Can you work these out from the model? Positions are in its coordinate system, mm. A direction names the side the tool comes from. Round coordinates to 2 decimals unless told otherwise and drop trailing zeros. Order: outer loops, then holes, each group sorted by start corner. A loop starts at its lowest first (then second) coordinate and runs counter-clockwise, first axis right, second up.
Q1. Will these pins go through, and if not, where does the flat tip stop? P1, Ø6.5, axis at x = 3.5, z = -13.5, coming from the +Y side; P2, Ø2.5, axis at x = 9.5, z = -7, coming from the +Y side.
Q2. We'd pull the mould along Y, two halves only. Please class faces 4 (the face through (8, 2, -13)), 5 (the face through (6.2, 3.8, -13)), 6 (the face through (27.88, 0.57, -0.6)), 7 (the face through (34, 7, -25.03)): pulls with the +Y half, pulls with the -Y half, needs draft (parallel to the pull), parting line crosses it, or undercut.
Q3. If I drill on line 1 (X direction, y = 2.5, z = -5.25); line 2 (X direction, y = 5, z = -21.25); line 3 (X direction, y = 7, z = -11.25), over which ranges is the centre line in solid material (lowest first)?
Q4. For faces 1 (the face through (12.4, 5, -13)), 2 (the face through (4, 5.6, -13)), 3 (the face through (0, 3, -13)), which set-ups out of +Z, -Z, +X, -X, +Y, -Y let a thin tool reach every point of the face, with its end or its side?
Q5. If we section it at C-C (x = 31.5): Please give me the cut outline in (y, z), plus the area to 3 significant figures.
Q6. If we section it at D-D (z = -19.5): Please give me the cut outline in (x, y), plus the area to 3 significant figures.
Q7. If we section it at A-A (y = 3): Please give me the cut outline in (x, z).
from build123d import *

# Parameters (mm, degrees)
SKETCH1_W           = 55
SKETCH1_H           = 25.6
BOSS_EXTRUDE1_DEPTH = 7.6
CUT_EXTRUDE1_DEPTH  = 25.6
FILLET1_R           = 2


with BuildPart() as part:
    # Sketch1 → Boss-Extrude1 (new body)
    with BuildSketch(Plane(origin=(0, 0, 0), x_dir=(1, 0, 0), z_dir=(0, 1, 0))):
        with Locations((27.5, 12.8)):
            Rectangle(SKETCH1_W, SKETCH1_H)
    extrude(amount=BOSS_EXTRUDE1_DEPTH)

    # Sketch2 → Cut-Extrude1 (cut)
    with BuildSketch(Plane(origin=(0, 0, -25.6), x_dir=(-1, 0, 0), z_dir=(0, 0, -1))):
        Polygon((-8, 5.6), (-4.4, 2), (-12.4, 2), (-12.4, 7.6), (0, 7.6), (0, 5.6), align=None)
    extrude(amount=-CUT_EXTRUDE1_DEPTH, mode=Mode.SUBTRACT)

    # Fillet1
    fillet1_edges = [part.edges().sort_by_distance(p)[0] for p in [
        (33.7, 7.6, -25.6),
        (33.7, 7.6, 0),
        (27.5, 0, -25.6),
        (27.5, 0, 0),
    ]]
    fillet(fillet1_edges, radius=FILLET1_R - 0.0001)  # a hair under: the kernel refuses the full size


solid = part.part
Solution:
1. P1: stops at y = 5.6
1. P2: stops at y = 2
2. face 4: undercut
2. face 5: undercut
2. face 6: pulls with the -Y half
2. face 7: pulls with the +Y half
3. line 1: x = 0 to 4.9, 12.4 to 55
3. line 2: x = 0 to 7.4, 12.4 to 55
3. line 3: x = 12.4 to 55
4. face 1: +Z, -Z, +Y
4. face 2: +Z, -Z, -X, +Y
4. face 3: +Z, -Z, -X, +Y, -Y
5. outline: (0, -23.6) arc R2 ccw to (2, -25.6) - (5.6, -25.6) arc R2 ccw to (7.6, -23.6) - (7.6, -2) arc R2 ccw to (5.6, 0) - (2, 0) arc R2 ccw to (0, -2) - close
5. area: 191 mm2
6. outline: (0, 0) - (55, 0) - (55, 7.6) - (12.4, 7.6) - (12.4, 2) - (4.4, 2) - (8, 5.6) - (0, 5.6) - close
6. area: 371 mm2
7. outline: (0, -25.6) - (5.4, -25.6) - (5.4, 0) - (0, 0) - close; (12.4, -25.6) - (55, -25.6) - (55, 0) - (12.4, 0) - close
